Part model, mm, in its own coordinate system. A direction names the side the tool comes from. Coordinates: 2 decimals unless noted, no trailing zeros. Order: outer loops, then holes, each group sorted by start corner. A loop starts at its lowest first (then second) coordinate and runs counter-clockwise, first axis right, second up.
```python
from build123d import *

# Parameters (mm, degrees)
EXTRUDE_1_DEPTH          = 8
CUT_EXTRUDE_1_REACH      = 61.933
SKETCH_2_R               = 1.5
EXTRUDE_2_DEPTH          = 22
CUT_EXTRUDE_2_DEPTH      = 22
EXTRUDE_3_DEPTH          = 9.5
SKETCH_8_R               = 1.5
CUT_EXTRUDE_3_DEPTH      = 5
SKETCH_10_R              = 2.5
CUT_EXTRUDE_4_DEPTH      = 2.5
SKETCH_11_R              = 1.5
EXTRUDE_4_DEPTH          = 1.25
SKETCH_12_R              = 1
EXTRUDE_5_DEPTH          = 1.95
FILLET_3_R               = 5
SKETCH_13_R              = 12.5
EXTRUDE_6_DEPTH          = 2
SKETCH_14_R              = 2.5
EXTRUDE_7_DEPTH          = 11
CUT_EXTRUDE_5_DEPTH      = 80.738572849
CUT_EXTRUDE_5_DEPTH_BACK = 9.8
EXTRUDE_6_2_DEPTH        = 5
EXTRUDE_8_REACH          = 61.412
SKETCH_18_W              = 1
SKETCH_18_H              = 1


with BuildPart() as part:
    # 草图1 → 凸台-拉伸1 (new body)
    with BuildSketch(Plane.XY):
        Polygon((0, 38), (4, 42), (38, 42), (42, 38), (42, 4), (38, 0), (4, 0), (0, 4), align=None)
    extrude(amount=-EXTRUDE_1_DEPTH)

    # 草图2 → 切除-拉伸1 (cut, up to next)
    with BuildSketch(Plane.XY, mode=Mode.PRIVATE) as cut_extrude_1_sk1:
        with Locations((5.5, 36.5)):
            Circle(SKETCH_2_R)
    cut_extrude_1_tool1 = extrude(cut_extrude_1_sk1.sketch, amount=-CUT_EXTRUDE_1_REACH, mode=Mode.PRIVATE) & part.part
    # 草图2 → 切除-拉伸1 (cut, up to next)
    with BuildSketch(Plane.XY, mode=Mode.PRIVATE) as cut_extrude_1_sk2:
        with Locations(Location((5.5, 5.5, 0), (0, 0, 180))):
            Circle(SKETCH_2_R)
    cut_extrude_1_tool2 = extrude(cut_extrude_1_sk2.sketch, amount=-CUT_EXTRUDE_1_REACH, mode=Mode.PRIVATE) & part.part
    # 草图2 → 切除-拉伸1 (cut, up to next)
    with BuildSketch(Plane.XY, mode=Mode.PRIVATE) as cut_extrude_1_sk3:
        with Locations(Location((36.5, 36.5, 0), (0, 0, 180))):
            Circle(SKETCH_2_R)
    cut_extrude_1_tool3 = extrude(cut_extrude_1_sk3.sketch, amount=-CUT_EXTRUDE_1_REACH, mode=Mode.PRIVATE) & part.part
    # 草图2 → 切除-拉伸1 (cut, up to next)
    with BuildSketch(Plane.XY, mode=Mode.PRIVATE) as cut_extrude_1_sk4:
        with Locations((36.5, 5.5)):
            Circle(SKETCH_2_R)
    cut_extrude_1_tool4 = extrude(cut_extrude_1_sk4.sketch, amount=-CUT_EXTRUDE_1_REACH, mode=Mode.PRIVATE) & part.part
    add(cut_extrude_1_tool1.solids().sort_by_distance((5.5, 36.5, 0))[0], mode=Mode.SUBTRACT)
    add(cut_extrude_1_tool2.solids().sort_by_distance((5.5, 5.5, 0))[0], mode=Mode.SUBTRACT)
    add(cut_extrude_1_tool3.solids().sort_by_distance((36.5, 36.5, 0))[0], mode=Mode.SUBTRACT)
    add(cut_extrude_1_tool4.solids().sort_by_distance((36.5, 5.5, 0))[0], mode=Mode.SUBTRACT)

    # 草图5 → 凸台-拉伸2 (add)
    with BuildSketch(Plane.XY):
        Polygon((0, 4), (4, 0), (38, 0), (42, 4), (42, 38), (38, 42), (4, 42), (0, 38), align=None)
    extrude(amount=EXTRUDE_2_DEPTH)

    # 草图6 → 切除-拉伸2 (cut)
    with BuildSketch(Plane.XY.offset(22)):
        Polygon((8, 0), (0, 8), (0, 4), (4, 0), align=None)
        Polygon((42, 8), (34, 0), (38, 0), (42, 4), align=None)
        Polygon((38, 42), (34, 42), (42, 34), (42, 38), align=None)
        Polygon((0, 38), (0, 34), (8, 42), (4, 42), align=None)
    extrude(amount=-CUT_EXTRUDE_2_DEPTH, mode=Mode.SUBTRACT)

    # 草图7 → 凸台-拉伸3 (add)
    with BuildSketch(Plane.XY.offset(22)):
        Polygon((0, 38), (0, 4), (4, 0), (38, 0), (42, 4), (42, 38), (38, 42), (4, 42), align=None)
    extrude(amount=EXTRUDE_3_DEPTH)

    # 草图8 → 切除-拉伸3 (cut)
    with BuildSketch(Plane.XY.offset(31.5)):
        with Locations((11.475, 21)):
            Circle(SKETCH_8_R)
        with Locations(Location((30.525, 21, 0), (0, 0, 180))):
            Circle(SKETCH_8_R)
    extrude(amount=-CUT_EXTRUDE_3_DEPTH, mode=Mode.SUBTRACT)

    # 草图10 → 切除-拉伸4 (cut)
    with BuildSketch(Plane.XY.offset(31.5)):
        with Locations((21, 21)):
            Circle(SKETCH_10_R)
    extrude(amount=-CUT_EXTRUDE_4_DEPTH, mode=Mode.SUBTRACT)

    # 草图11 → 凸台-拉伸4 (add)
    with BuildSketch(Plane.XY.offset(29)):
        with Locations((21, 21)):
            Circle(SKETCH_11_R)
    extrude(amount=EXTRUDE_4_DEPTH)

    # 草图12 → 凸台-拉伸5 (add)
    with BuildSketch(Plane.XY.offset(30.25)):
        with Locations((21, 21)):
            Circle(SKETCH_12_R)
    extrude(amount=EXTRUDE_5_DEPTH)

    # 圆角3
    fillet_3_edges = [part.edges().sort_by_distance(p)[0] for p in [
        (42, 8, 11),
        (34, 0, 11),
        (0, 8, 11),
        (8, 0, 11),
        (0, 34, 11),
        (8, 42, 11),
        (42, 34, 11),
        (34, 42, 11),
    ]]
    fillet(fillet_3_edges, radius=FILLET_3_R)

    # 草图13 → Extrude 6 (add)
    with BuildSketch(Plane(origin=(0, 0, -8), x_dir=(-1, 0, 0), z_dir=(0, 0, -1))):
        with Locations((-21, 21)):
            Circle(SKETCH_13_R)
    extrude(amount=EXTRUDE_6_DEPTH)

    # 草图14 → 凸台-拉伸7 (add)
    with BuildSketch(Plane(origin=(0, 0, -10), x_dir=(-1, 0, 0), z_dir=(0, 0, -1))):
        with Locations(Location((-21, 21, 0), (0, 0, 180))):
            Circle(SKETCH_14_R)
    extrude(amount=EXTRUDE_7_DEPTH)

    # 草图16 → 切除-拉伸5 (cut, two sides: drawn at the far end of the back side and taken through both)
    with BuildSketch(Plane(origin=(0, 0, -21), x_dir=(-1, 0, 0), z_dir=(0, 0, -1)).offset(-CUT_EXTRUDE_5_DEPTH_BACK)):
        Polygon((-96.850602173, 23), (-22.5, 23), (-19.5, 23), (54.850602173, 23), (54.850602173, 171.701204346), (-96.850602173, 171.701204346), align=None)
    extrude(amount=CUT_EXTRUDE_5_DEPTH + CUT_EXTRUDE_5_DEPTH_BACK, mode=Mode.SUBTRACT)

    # 草图17 → Extrude 6 2 (add)
    with BuildSketch(Plane.ZY):
        Polygon((27, 15), (27, 12.5), (32, 12.5), (32, 29.5), (27, 29.5), (27, 27), (28, 27), (28, 28.5), (31, 28.5), (31, 13.5), (28, 13.5), (28, 15), align=None)
    extrude(amount=EXTRUDE_6_2_DEPTH)

    # 草图18 → 凸台-拉伸8 (add, up to next)
    with BuildSketch(Plane(origin=(0, 15, 0), x_dir=(1, 0, 0), z_dir=(0, 1, 0)), mode=Mode.PRIVATE) as extrude_8_sk1:
        with Locations((-0.5, -27.5)):
            Rectangle(SKETCH_18_W, SKETCH_18_H)
    extrude_8_tool1 = extrude(extrude_8_sk1.sketch, amount=EXTRUDE_8_REACH, mode=Mode.PRIVATE) - part.part
    add(extrude_8_tool1.solids().sort_by_distance((-0.5, 15, 27.5))[0])


solid = part.part
```
(1) Slice it at C-C, the plane z = 12. Give the cut face in (x, y), then the cut area to 3 significant figures.
(2) Pull direction Y, two halves, no side cores. Call faces 6 (the face through (-2, 21, 32)), 7 (the face through (-2, 13.5, 30)), 8 (the face through (41.63, 8.18, 10.85)): +Y half, -Y half, draft (parallel to the pull), parting line (faces both ways), or undercut.
(3) Tool access for faces 1 (the face through (38, 4, 11)), 2 (the face through (8.13, 0.39, 10.85)), 3 (the face through (21, 20, 31)), 4 (the face through (-0.3, 20.9, 28)), 5 (the face through (5, 37, 0)): list every direction of +Z, -Z, +X, -X, +Y, -Y with a clear straight run to the whole face (end or side of a thin tool).
(4) Slice it at B-B, the plane x = 21. Give the cut face in (y, z), then the cut area to 3 significant figures.
(5) Probe line 1 (Y direction, x = 21, z = 30.85); line 2 (Y direction, x = 36.5, z = -1.5); line 3 (Z direction, x = 5, y = 40). List the from-to ranges inside material, lowest first.
(6) Drop flat-ended pins along their axis: pin 1 (5.5 mm diameter, centred on x = -1.5, z = 28.5, fed in from -Y); pin 2 (2 mm diameter, centred on x = 25.5, y = 5.5, fed in from -Z); pin 3 (1.1 mm diameter, centred on x = -4, z = 27.5, fed in from -Y). Give the stop position or say it passes through.
(7) Slice it at A-A, the plane y = 5.5. Give the cut face in (x, z), then the cut area to 3 significant figures.
Here are the results:
1. outline: (0, 10.07) arc R5 ccw to (1.46, 6.54) - (6.54, 1.46) arc R5 ccw to (10.07, 0) - (31.93, 0) arc R5 ccw to (35.46, 1.46) - (40.54, 6.54) arc R5 ccw to (42, 10.07) - (42, 31.93) arc R5 ccw to (40.54, 35.46) - (35.46, 40.54) arc R5 ccw to (31.93, 42) - (10.07, 42) arc R5 ccw to (6.54, 40.54) - (1.46, 35.46) arc R5 ccw to (0, 31.93) - close
1. area: 1,630 mm2
2. face 6: draft
2. face 7: undercut
2. face 8: -Y half
3. face 1: +X, -Y
3. face 2: -X, -Y
3. face 3: +Z
3. face 4: -X
3. face 5: -Z
4. outline: (0, -8) - (8.5, -8) - (8.5, -10) - (18.5, -10) - (18.5, -21) - (23, -21) - (23, -11.2) - (23.5, -11.2) - (23.5, -10) - (33.5, -10) - (33.5, -8) - (42, -8) - (42, 31.5) - (23.5, 31.5) - (23.5, 29) - (22.5, 29) - (22.5, 30.25) - (22, 30.25) - (22, 32.2) - (20, 32.2) - (20, 30.25) - (19.5, 30.25) - (19.5, 29) - (18.5, 29) - (18.5, 31.5) - (0, 31.5) - close
4. area: 1,750 mm2
5. line 1: y = 0 to 18.5, 20 to 22, 23.5 to 42
5. line 2: y = 0 to 4, 7 to 35, 38 to 42
5. line 3: z = -8 to 0, 22 to 31.5
6. pin 1: stops at y = 2.75
6. pin 2: stops at z = -8
6. pin 3: stops at y = 12.5
7. outline: (0, -8) - (4, -8) - (4, 0) - (7, 0) - (7, -8) - (35, -8) - (35, 0) - (38, 0) - (38, -8) - (42, -8) - (42, 0) - (39.5, 0) - (39.5, 22) - (42, 22) - (42, 31.5) - (0, 31.5) - (0, 22) - (2.5, 22) - (2.5, 0) - (0, 0) - close
7. area: 1,500 mm2
